Source: CAD feature listing. Evaluate the final solid. Frame: model axes, mm. Round coordinates to 2 decimals unless told otherwise and drop trailing zeros. Loops run counter-clockwise (first coordinate to the right, second up) from the corner with the lowest first, then second, coordinate; pieces in that order, holes last. Notation, with made-up numbers: M 47,62 L 73,62 A13 ccw 73,70 Z; hole C 55,34.5 d11. An arc over 180 degrees is marked long. One line per item, written item: value.
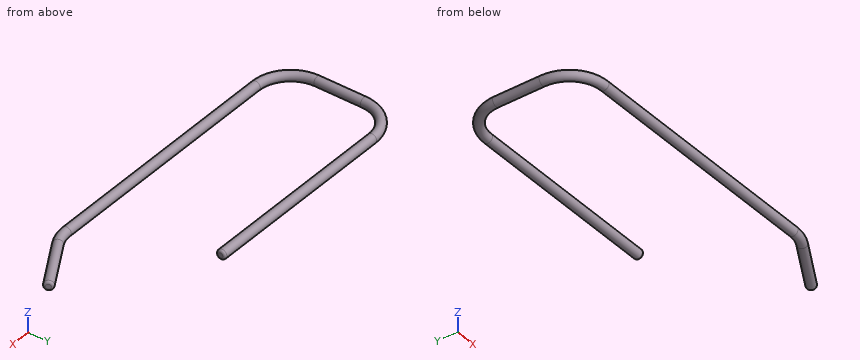
from build123d import *

# Parameters (mm, degrees)
SWEEP1_PROFILE_R = 4
FILLET1_R        = 2


with BuildPart() as part:
    # Sweep1: sweep along a path in Sketch1
    with BuildLine(Plane.XY) as sweep1_path:
        Line((150, -71.132486541), (106.961524227, -95.980762114))
        ThreePointArc((106.961524227, -95.980762114), (99.72609558, -98.977774789), (91.961524227, -100))
        Line((91.961524227, -100), (-120, -100))
        ThreePointArc((-120, -100), (-141.213203436, -91.213203436), (-150, -70))
        Line((-150, -70), (-150, -30))
        ThreePointArc((-150, -30), (-141.213203436, -8.786796564), (-120, 0))
        Line((-120, 0), (0, 0))
        Line((0, 0), (50, 0))
    # Sweep1 profile (on start of the path) → Sweep1 (sweep)
    with BuildSketch(Plane(origin=(150, -71.132486541, 0), x_dir=(0.5, -0.866025404, 0), z_dir=(-0.866025404, -0.5, 0))):
        Circle(SWEEP1_PROFILE_R)
    sweep(path=sweep1_path.line)

    # Fillet1
    fillet1_edges = [part.edges().sort_by_distance(p)[0] for p in [
        (148, -67.668384925, 0),
        (50, -4, 0),
    ]]
    fillet(fillet1_edges, radius=FILLET1_R)


solid = part.part
1. Pin query (flat end, axial travel): pin 1 (2 mm diameter, centred on x = -42.5, z = -1.5, fed in from +Y); pin 2 (2 mm diameter, centred on x = -30.5, z = 1.5, fed in from -Y); pin 3 (1 mm diameter, centred on y = -69.5, z = -2, fed in from +X). Return the tip coordinate at first contact, or that it passes through.
Report:
pin 1: stops at y = 3.97
pin 2: stops at y = -103.97
pin 3: stops at x = 149.31
2. Ray query, line 1 (X direction, y = -33.5, z = 0); line 2 (Y direction, x = -7, z = -2); line 3 (Y direction, x = 28.5, z = 2.75). Return the intervals inside material, ascending. Write a range as [from, to].
Report:
line 1: x = [-154, -146]
line 2: y = [-103.46, -96.54], [-3.46, 3.46]
line 3: y = [-102.9, -97.1], [-2.9, 2.9]
3. Section query B-B (y = -53.5). Return the cut outline in (x, z), and give its area (3 significant figures).
Report:
outline: C -150,0 d8
area: 50.3 mm2
4. Section query A-A (x = -38.5). Return the cut outline in (y, z).
Report:
outline: C -100,0 d8; C 0,0 d8
5. Section query C-C (x = 84). Return the cut outline in (y, z), and give its area (3 significant figures).
Report:
outline: C -100,0 d8
area: 50.3 mm2
